Here's the drawing with two shaded views (mm, measured from the low corner). I have some questions. A direction names the side the tool comes from. Coordinates: 2 decimals unless noted, no trailing zeros. Write each loop counter-clockwise with the first axis right and the second up, starting at its lowest first coordinate (ties: lowest second). Pieces come first, ordered by that corner, then holes. Notation, with made-up numbers: (45.25, 73) - (69.25, 73) arc R21 cw to (69.25, 102) - close; hole circle Ø3 at (-20.5, 32). An arc over 180 degrees is marked (long way). Answer in a Markdown table with one row per item. Add a question column.
Item 1: I'm going to push flat-ended pins straight in: pin 1 (4 mm diameter, centred on x = 4, y = 15, fed in from -Z); pin 2 (1.9 mm diameter, centred on x = 12.7, y = 12.7, fed in from +Z). Where does each tip first touch, or does it pass through?
Item 2: If I drill on probe 1 along Z at (x, y) = (21, 1.5) (3 decimals); probe 2 along Y at (x, z) = (1.1, 12.7), over which ranges is the centre line in solid material (lowest first)? Write a range as from..to.
Item 3: Imagine slicing it at C-C (z = 17). Please give me the cut outline in (x, y) (3 decimals), plus the area to 3 significant figures.
Item 4: Imagine slicing it at D-D (z = 12.7). Please give me the cut outline in (x, y) (1 decimal), plus the area to 3 significant figures.
Item 5: We'd pull the mould along Z, two halves only. Please class the marked faces 1, 2 and 3: +Z half, -Z half, draft (parallel to the pull), parting line (faces both ways), or undercut.
Item 6: Imagine slicing it at B-B (y = 15). Please give me the cut outline in (x, z) (3 decimals).
Item 7: Which directions (+Z, -Z, +X, -X, +Y, -Y) give clear straight access to the entire face, cutting with the end or side of a thin tool? Please do the marked faces 4 and 5.
Item 8: Imagine slicing it at A-A (x = 12.7). Please give me the cut outline in (y, z) (1 decimal).
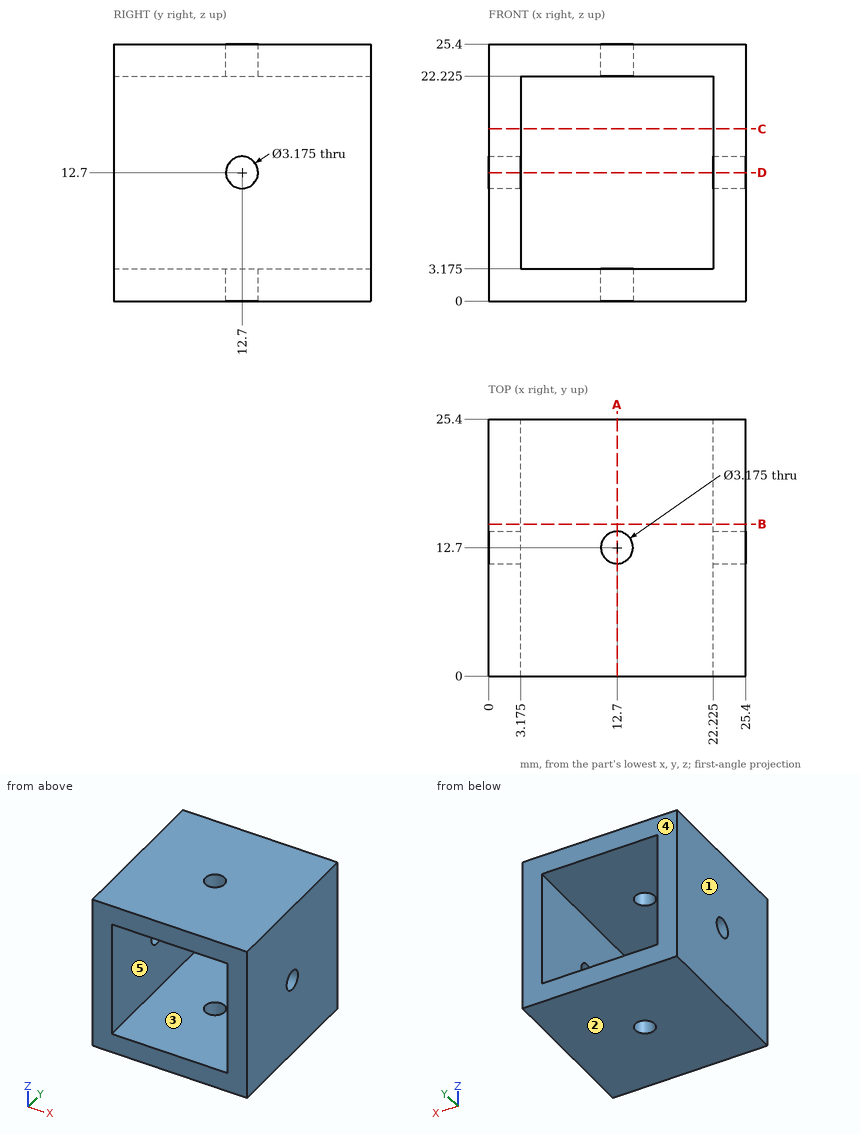
Here are the results:
| question | item | result |
|---|---|---|
| 1 | pin 1 | stops at z = 0 |
| 1 | pin 2 | passes through |
| 2 | probe 1 | z = 0..3.175, 22.225..25.4 |
| 2 | probe 2 | y = 0..11.11, 14.29..25.4 |
| 3 | outline | (0, 0) - (3.175, 0) - (3.175, 25.4) - (0, 25.4) - close; (22.225, 0) - (25.4, 0) - (25.4, 25.4) - (22.225, 25.4) - close |
| 3 | area | 161 mm2 |
| 4 | outline | (0, 0) - (3.2, 0) - (3.2, 11.1) - (0, 11.1) - close; (0, 14.3) - (3.2, 14.3) - (3.2, 25.4) - (0, 25.4) - close; (22.2, 0) - (25.4, 0) - (25.4, 11.1) - (22.2, 11.1) - close; (22.2, 14.3) - (25.4, 14.3) - (25.4, 25.4) - (22.2, 25.4) - close |
| 4 | area | 141 mm2 |
| 5 | face 1 | draft |
| 5 | face 2 | -Z half |
| 5 | face 3 | undercut |
| 6 | outline | (0, 0) - (25.4, 0) - (25.4, 25.4) - (0, 25.4) - close; hole (3.175, 3.175) - (22.225, 3.175) - (22.225, 22.225) - (3.175, 22.225) - close |
| 7 | face 4 | +Z, -Z, +X, -X, +Y |
| 7 | face 5 | +Y, -Y |
| 8 | outline | (0, 0) - (11.1, 0) - (11.1, 3.2) - (0, 3.2) - close; (0, 22.2) - (11.1, 22.2) - (11.1, 25.4) - (0, 25.4) - close; (14.3, 0) - (25.4, 0) - (25.4, 3.2) - (14.3, 3.2) - close; (14.3, 22.2) - (25.4, 22.2) - (25.4, 25.4) - (14.3, 25.4) - close |
